CAD build for the part. Positions are in the model's coordinates, mm. Coordinates: 2 decimals unless noted, no trailing zeros. Loops run counter-clockwise (first coordinate to the right, second up) from the corner with the lowest first, then second, coordinate; pieces in that order, holes last. Notation, with made-up numbers: (9, 68) -> (57, 68) arc R30 ccw to (57, 103) -> close; hole circle Ø3 at (6.5, 63.5). An arc over 180 degrees is marked (long way). Return JSON: item names as keys, results as strings. Group by question number.
(1) Flat gauge pins, fed straight in: pin 1 Ø4 at (x, z) = (52.49, -27.45) entering from -Y; pin 2 Ø2.5 at (x, z) = (81.46, 0) entering from +Y; pin 3 Ø4.5 at (x, z) = (-52.37, 0) entering from +Y; pin 4 Ø5.5 at (x, z) = (0, 52.37) entering from -Y. Where does each tip first touch, or does it go through?
(2) Saw through at A-A on z = 0. Write the cut outline in (x, y) (3 decimals).
(3) Saw through at B-B on x = 0. Write the cut outline in (y, z) (3 decimals), then the cut area to 3 significant figures.
(4) Probe L1, parallel to X at y = -1.5, z = 0; L2, parallel to X at y = -2.3, z = 3.5; L3, parallel to X at y = -2.35, z = -29.5. List the from-to ranges inside material, lowest first.
(5) Mould opens along Z. For faces 1 (the face through (-1, -1, 51)), 2 (the face through (86.23, -1.57, -0.26)), 3 (the face through (16, 0, -14)), 4 (the face through (-35.375, -0.768, -36.666)) say: pulls with the +Z half, pulls with the -Z half, needs draft (parallel to the pull), parting line crosses it, or undercut.
(6) Saw through at C-C on y = -2.35. Give the number of separate pieces and of enclosed holes in the cut face, then the cut area to 3 significant figures.
(7) Saw through at D-D on x = 16. Write the cut outline in (y, z) (3 decimals).
```python
from build123d import *

# Parameters (mm, degrees)
SKETCH1_R                    = 57.15
SKETCH1_R_2                  = 20
BOSS_EXTRUDE1_DEPTH          = 3.175
BOSS_EXTRUDE2_START          = -3.175
BOSS_EXTRUDE2_DEPTH          = 3.175
CSK_FOR_M3_SFHCS1_AT_2_COUNT = 2
CSK_FOR_M3_SFHCS1_AT_2_PITCH = 74.069152487
CSK_FOR_M3_SFHCS1_AT_3_COUNT = 2
CSK_FOR_M3_SFHCS1_AT_3_PITCH = 96.776011479
CSK_FOR_M3_SFHCS1_AT_4_COUNT = 2
CSK_FOR_M3_SFHCS1_AT_4_PITCH = 104.7496
CSK_FOR_M3_SFHCS1_AT_5_COUNT = 2
CSK_FOR_M3_SFHCS1_AT_5_PITCH = 95.534640107
CSK_FOR_M3_SFHCS1_AT_6_COUNT = 2
CSK_FOR_M3_SFHCS1_AT_6_PITCH = 96.842619006
CSK_FOR_M3_SFHCS1_AT_7_COUNT = 2
CSK_FOR_M3_SFHCS1_AT_7_PITCH = 58.10838136
CSK_FOR_M3_SFHCS1_AT_8_COUNT = 2
CSK_FOR_M3_SFHCS1_AT_8_PITCH = 40.085936467


with BuildPart() as part:
    # Sketch1 → Boss-Extrude1 (new body)
    with BuildSketch(Plane(origin=(0, 0, 0), x_dir=(1, 0, 0), z_dir=(0, 1, 0))):
        with Locations(Location((0, 0, 0), (0, 0, 270))):
            Circle(SKETCH1_R)
        with Locations(Location((0, 0, 0), (0, 0, 270))):
            Circle(SKETCH1_R_2, mode=Mode.SUBTRACT)
    extrude(amount=-BOSS_EXTRUDE1_DEPTH)

    # Sketch2 → Boss-Extrude2 (add)
    with BuildSketch(Plane(origin=(0, -3.175, 0), x_dir=(-1, 0, 0), z_dir=(0, -1, 0)).offset(BOSS_EXTRUDE2_START)):
        with BuildLine():
            Line((-32.41020794, 47.071232418), (-77.986402647, 15.690410806))
            ThreePointArc((-77.986402647, 15.690410806), (-86.233, 0), (-77.986402647, -15.690410806))
            Line((-77.986402647, -15.690410806), (-32.41020794, -47.071232418))
            ThreePointArc((-32.41020794, -47.071232418), (-57.15, 0), (-32.41020794, 47.071232418))
        make_face()
    extrude(amount=BOSS_EXTRUDE2_DEPTH)

    # Sketch7 → CSK for M3 SFHCS1 (revolve, cut)
    with BuildSketch(Plane(origin=(0, -3.175, 52.3748), x_dir=(0, 0, -1), z_dir=(1, 0, 0))):
        Polygon((0, 0), (0, 3.175), (1.7, 3.175), (1.7, 1.66), (3.36, 0), align=None)
    csk_for_m3_sfhcs1 = revolve(axis=Axis((0, -9.525, 52.3748), (0, 1, 0)), mode=Mode.SUBTRACT)

    # CSK for M3 SFHCS1 at 2: CSK for M3 SFHCS1 ×2
    with Locations(*[Vector(-0.7071067811865477, 0, -0.7071067811865475) * (i * CSK_FOR_M3_SFHCS1_AT_2_PITCH) for i in range(1, CSK_FOR_M3_SFHCS1_AT_2_COUNT)]):
        add(csk_for_m3_sfhcs1, mode=Mode.SUBTRACT)

    # CSK for M3 SFHCS1 at 3: CSK for M3 SFHCS1 ×2
    with Locations(*[Vector(-0.3826834323650908, 0, -0.9238795325112864) * (i * CSK_FOR_M3_SFHCS1_AT_3_PITCH) for i in range(1, CSK_FOR_M3_SFHCS1_AT_3_COUNT)]):
        add(csk_for_m3_sfhcs1, mode=Mode.SUBTRACT)

    # CSK for M3 SFHCS1 at 4: CSK for M3 SFHCS1 ×2
    with Locations(*[(0, 0, -i * CSK_FOR_M3_SFHCS1_AT_4_PITCH) for i in range(1, CSK_FOR_M3_SFHCS1_AT_4_COUNT)]):
        add(csk_for_m3_sfhcs1, mode=Mode.SUBTRACT)

    # CSK for M3 SFHCS1 at 5: CSK for M3 SFHCS1 ×2
    with Locations(*[Vector(0.5494368566637676, 0, -0.8355352419493978) * (i * CSK_FOR_M3_SFHCS1_AT_5_PITCH) for i in range(1, CSK_FOR_M3_SFHCS1_AT_5_COUNT)]):
        add(csk_for_m3_sfhcs1, mode=Mode.SUBTRACT)

    # CSK for M3 SFHCS1 at 6: CSK for M3 SFHCS1 ×2
    with Locations(*[Vector(0.84113586390326, 0, -0.5408238700868485) * (i * CSK_FOR_M3_SFHCS1_AT_6_PITCH) for i in range(1, CSK_FOR_M3_SFHCS1_AT_6_COUNT)]):
        add(csk_for_m3_sfhcs1, mode=Mode.SUBTRACT)

    # CSK for M3 SFHCS1 at 7: CSK for M3 SFHCS1 ×2
    with Locations(*[Vector(0.9033163742395407, 0, -0.42897497366481663) * (i * CSK_FOR_M3_SFHCS1_AT_7_PITCH) for i in range(1, CSK_FOR_M3_SFHCS1_AT_7_COUNT)]):
        add(csk_for_m3_sfhcs1, mode=Mode.SUBTRACT)

    # CSK for M3 SFHCS1 at 8: CSK for M3 SFHCS1 ×2
    with Locations(*[Vector(-0.9238795325112864, 0, -0.3826834323650906) * (i * CSK_FOR_M3_SFHCS1_AT_8_PITCH) for i in range(1, CSK_FOR_M3_SFHCS1_AT_8_COUNT)]):
        add(csk_for_m3_sfhcs1, mode=Mode.SUBTRACT)


solid = part.part
```
Geometry results:
{
 "1": {"pin 1": "y = -1.82", "pin 2": "through", "pin 3": "y = 0", "pin 4": "y = -2.57"},
 "2": {"outline": "(-57.15, -3.175) -> (-55.735, -3.175) -> (-54.075, -1.515) -> (-54.075, 0) -> (-57.15, 0) -> close; (-50.675, -1.515) -> (-49.015, -3.175) -> (-20, -3.175) -> (-20, 0) -> (-50.675, 0) -> close; (20, -3.175) -> (78.098, -3.175) -> (79.758, -1.515) -> (79.758, 0) -> (20, 0) -> close; (83.158, -1.515) -> (84.818, -3.175) -> (86.233, -3.175) -> (86.233, 0) -> (83.158, 0) -> close"},
 "3": {"outline": "(-3.175, -57.15) -> (0, -57.15) -> (0, -54.075) -> (-1.515, -54.075) -> (-3.175, -55.735) -> close; (-3.175, -49.015) -> (-1.515, -50.675) -> (0, -50.675) -> (0, -20) -> (-3.175, -20) -> close; (-3.175, 20) -> (0, 20) -> (0, 50.675) -> (-1.515, 50.675) -> (-3.175, 49.015) -> close; (-3.175, 55.735) -> (-1.515, 54.075) -> (0, 54.075) -> (0, 57.15) -> (-3.175, 57.15) -> close", "area": "209 mm²"},
 "4": {"L1": "-57.15 to -54.07, -50.67 to -20, 20 to 79.76, 83.16 to 86.23", "L2": "-57.04 to -19.69, 19.69 to 85.91", "L3": "-48.95 to 51, 53.98 to 57.93"},
 "5": {"face 1": "undercut", "face 2": "parting line crosses it", "face 3": "needs draft", "face 4": "undercut"},
 "6": {"separate pieces": "1", "enclosed holes": "9", "area": "10,200 mm²"},
 "7": {"outline": "(-3.175, -54.865) -> (0, -54.865) -> (0, -12) -> (-3.175, -12) -> close; (-3.175, 12) -> (0, 12) -> (0, 54.865) -> (-3.175, 54.865) -> close"}
}
